from build123d import *

# Parameters (mm, degrees)
F0_W     = 38.1
F0_H     = 25.4
F1_DEPTH = 12.7
F2_W     = 34.925
F2_H     = 22.225
F3_DEPTH = 1.5875
F4_R     = 0.762
F5_R     = 0.254
F6_W     = 7.1628
F6_H     = 2.032
F7_DEPTH = 25.4


with BuildPart() as f1:
    # F0 (on Top) → F1 (new body)
    with BuildSketch(Plane.XY):
        Rectangle(F0_W, F0_H)
    extrude(amount=F1_DEPTH)

    # F2 (on face) → F3 (cut)
    with BuildSketch(Plane.XY.offset(12.7)):
        Rectangle(F2_W, F2_H)
    extrude(amount=-F3_DEPTH, mode=Mode.SUBTRACT)

    # F4
    f4_edges = [f1.edges().sort_by_distance(p)[0] for p in [
        (-19.05, -12.7, 6.35),
        (-19.05, 12.7, 6.35),
        (19.05, 12.7, 6.35),
        (19.05, -12.7, 6.35),
    ]]
    fillet(f4_edges, radius=F4_R)

    # F5
    f5_edges = [f1.edges().sort_by_distance(p)[0] for p in [
        (0, 12.7, 12.7),
        (18.826815, 12.476815, 12.7),
        (-18.826815, 12.476815, 12.7),
        (19.05, 0, 12.7),
        (-19.05, 0, 12.7),
        (18.826815, -12.476815, 12.7),
        (-18.826815, -12.476815, 12.7),
        (0, -12.7, 12.7),
        (0, 11.1125, 12.7),
        (-17.4625, 0, 12.7),
        (0, -11.1125, 12.7),
        (17.4625, 0, 12.7),
    ]]
    fillet(f5_edges, radius=F5_R)

    # F6 (on Top) → F7 (cut)
    with BuildSketch(Plane.XY):
        with Locations((-10.7061, -7.62)):
            Rectangle(F6_W, F6_H)
        with Locations((-9.91108, 0)):
            Rectangle(F6_W, F6_H)
        with Locations((-8.32358, 7.62)):
            Rectangle(F6_W, F6_H)
        with Locations((9.13892, 0)):
            Rectangle(F6_W, F6_H)
        with Locations((8.3439, -7.62)):
            Rectangle(F6_W, F6_H)
        with Locations((10.72642, 7.62)):
            Rectangle(F6_W, F6_H)
    extrude(amount=F7_DEPTH, mode=Mode.SUBTRACT)


solid = f1.part
Could you check a few things on this model? Use its own coordinates, in mm. A direction names the side the tool comes from. Coordinates: 2 decimals unless noted, no trailing zeros. Loops run counter-clockwise (first coordinate to the right, second up) from the corner with the lowest first, then second, coordinate; pieces in that order, holes last. Notation, with made-up numbers: (73, -1.5) -> (121, -1.5) arc R14 cw to (121, 23.5) -> close; hole circle Ø9 at (-16, 87.5). An arc over 180 degrees is marked (long way). Answer in a Markdown table with one row per item.
(1) Thinking about a two-plate mould opening in Y: for faces 1 (the face through (19.05, 0, 6)), 2 (the face through (0, 12.7, 6)), 3 (the face through (-11.905, 8, 5)), which applies, released by +Y, released by -Y, zero draft, split by the parting line, or undercut?
Results found:
| item | result |
|---|---|
| face 1 | zero draft |
| face 2 | released by +Y |
| face 3 | undercut |
(2) Will this pin go through, and if not, where does the flat tip stop? pin 1 Ø3 at (x, y) = (-14, -6) entering from +Z.
Results found:
| item | result |
|---|---|
| pin 1 | stops at z = 11.11 |
(3) Imagine slicing it at D-D (x = 8.5). List the corners of the cut face in (y, z) for me.
Results found:
| item | result |
|---|---|
| outline | (-12.7, 0) -> (-8.64, 0) -> (-8.64, 11.11) -> (-11.11, 11.11) -> (-11.11, 12.45) arc R0.25 ccw to (-11.37, 12.7) -> (-12.45, 12.7) arc R0.25 ccw to (-12.7, 12.45) -> close; (-6.6, 0) -> (-1.02, 0) -> (-1.02, 11.11) -> (-6.6, 11.11) -> close; (1.02, 0) -> (6.6, 0) -> (6.6, 11.11) -> (1.02, 11.11) -> close; (8.64, 0) -> (12.7, 0) -> (12.7, 12.45) arc R0.25 ccw to (12.45, 12.7) -> (11.37, 12.7) arc R0.25 ccw to (11.11, 12.45) -> (11.11, 11.11) -> (8.64, 11.11) -> close |
(4) Imagine slicing it at A-A (x = -13). List the corners of the cut face in (y, z) for me.
Results found:
| item | result |
|---|---|
| outline | (-12.7, 0) -> (-8.64, 0) -> (-8.64, 11.11) -> (-11.11, 11.11) -> (-11.11, 12.45) arc R0.25 ccw to (-11.37, 12.7) -> (-12.45, 12.7) arc R0.25 ccw to (-12.7, 12.45) -> close; (-6.6, 0) -> (-1.02, 0) -> (-1.02, 11.11) -> (-6.6, 11.11) -> close; (1.02, 0) -> (12.7, 0) -> (12.7, 12.45) arc R0.25 ccw to (12.45, 12.7) -> (11.37, 12.7) arc R0.25 ccw to (11.11, 12.45) -> (11.11, 11.11) -> (1.02, 11.11) -> close |
(5) Imagine slicing it at B-B (z = 8.5). Give the number of separate pieces and of enclosed holes in the cut face, plus the area to 3 significant figures.
Results found:
| item | result |
|---|---|
| separate pieces | 1 |
| enclosed holes | 6 |
| area | 880 mm^2 |
(6) If I drill on probe 1 along Y at (x, z) = (6, 9); probe 2 along X at (y, z) = (-8.25, 1.5); probe 3 along Y at (x, z) = (12, 5.25), over which ranges is the centre line in solid material (lowest first)?
Results found:
| item | result |
|---|---|
| probe 1 | y = -12.7 to -8.64, -6.6 to -1.02, 1.02 to 12.7 |
| probe 2 | x = -19.05 to -14.29, -7.12 to 4.76, 11.93 to 19.05 |
| probe 3 | y = -12.7 to -1.02, 1.02 to 6.6, 8.64 to 12.7 |
(7) For faces 4 (the face through (17.462, 0, 12)), 5 (the face through (12.72, 0, 5)), which set-ups out of +Z, -Z, +X, -X, +Y, -Y let a thin tool reach every point of the face, with its end or its side?
Results found:
| item | result |
|---|---|
| face 4 | +Z |
| face 5 | +Z, -Z |
(8) Imagine slicing it at C-C (y = -2.75). List the corners of the cut face in (x, z) for me.
Results found:
| item | result |
|---|---|
| outline | (-19.05, 0) -> (19.05, 0) -> (19.05, 12.45) arc R0.25 ccw to (18.8, 12.7) -> (17.72, 12.7) arc R0.25 ccw to (17.46, 12.45) -> (17.46, 11.11) -> (-17.46, 11.11) -> (-17.46, 12.45) arc R0.25 ccw to (-17.72, 12.7) -> (-18.8, 12.7) arc R0.25 ccw to (-19.05, 12.45) -> close |
